The drawing under review shows one solid part. Ordinate dimensions are in mm from its lowest x, y, z. A direction names the side the tool comes from. Coordinates: 2 decimals unless noted, no trailing zeros. Write each loop counter-clockwise with the first axis right and the second up, starting at its lowest first coordinate (ties: lowest second). Pieces come first, ordered by that corner, then holes.
Q1. Add section C-C, the plane x = 5.5. Give the boundary of the cut face in (y, z), plus the area to 3 significant figures.
Q2. The part is to be moulded in two halves that separate along Z. For the marked faces 3, 4 and 5, say which applies: +Z half, -Z half, draft (parallel to the pull), parting line (faces both ways), or undercut.
Q3. Add section A-A, the plane z = 9. Give the boundary of the cut face in (x, y), plus the area to 3 significant figures.
Q4. Clearance check with flat-ended pins moving along their axes: pin 1 Ø3 at (x, y) = (6, 4) entering from +Z; pin 2 Ø2.5 at (y, z) = (9, 14.95) entering from +X; pin 3 Ø6.5 at (y, z) = (14.95, 9) entering from +X. State where each tip first meets the part, or that it passes through.
Q5. Add section D-D, the plane x = 1.25. Give the boundary of the cut face in (y, z).
Q6. Machinability: for the marked faces 1 and 2, which of the approach directions +Z, -Z, +X, -X, +Y, -Y give a long, thin tool a straight path to every point of the face, cutting with its end or side? Answer none if there is none.
Q7. To check wall thickness, follow probe 1 along Y at (x, z) = (5.75, 7.25); probe 2 along Z at (x, y) = (2.5, 10.25); probe 3 along Z at (x, y) = (4, 8.5). State the ranges of each line that lie inside material, in increasing order.
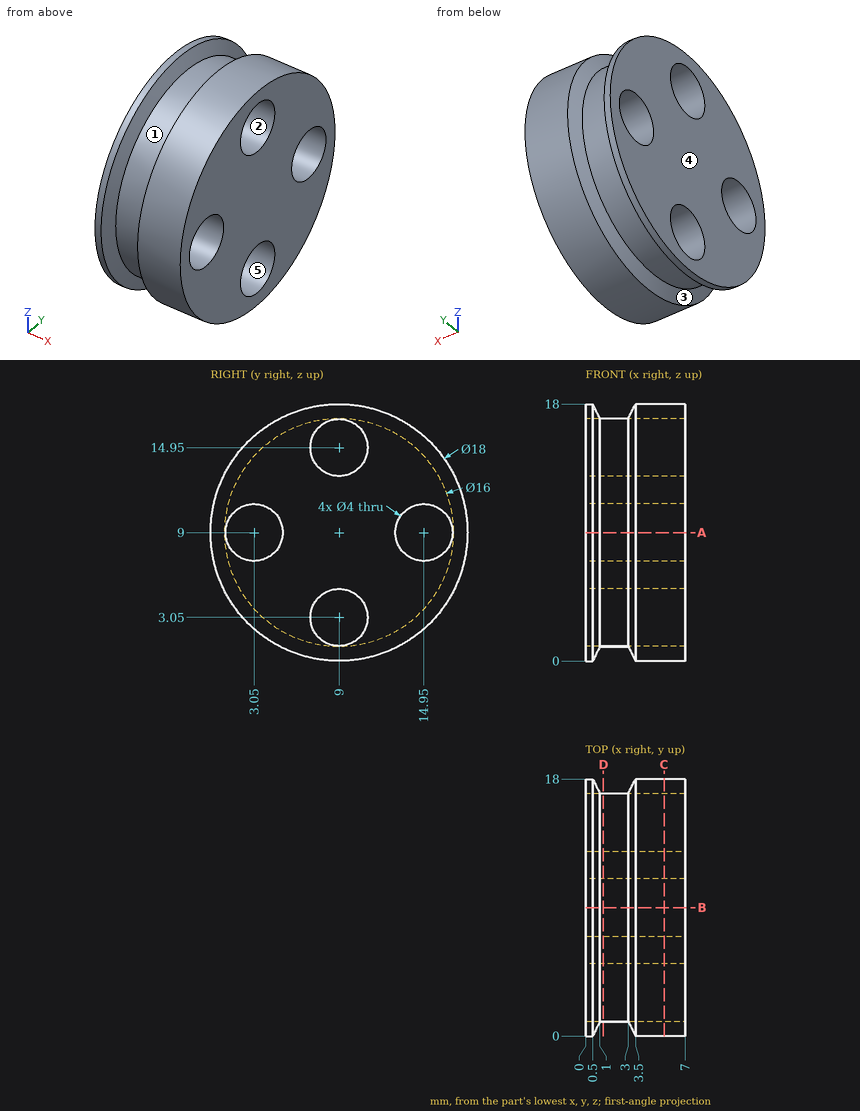
Here are the results:
1. outline: circle Ø18 at (9, 9); hole circle Ø4 at (3.05, 9); hole circle Ø4 at (9, 3.05); hole circle Ø4 at (9, 14.95); hole circle Ø4 at (14.95, 9)
1. area: 204 mm2
2. face 3: parting line
2. face 4: draft
2. face 5: undercut
3. outline: (0, 0) - (0.5, 0) - (1, 1) - (3, 1) - (3.5, 0) - (7, 0) - (7, 1.05) - (0, 1.05) - close; (0, 5.05) - (7, 5.05) - (7, 12.95) - (0, 12.95) - close; (0, 16.95) - (7, 16.95) - (7, 18) - (3.5, 18) - (3, 17) - (1, 17) - (0.5, 18) - (0, 18) - close
3. area: 65.0 mm2
4. pin 1: stops at z = 17.29
4. pin 2: passes through
4. pin 3: stops at x = 7
5. outline: circle Ø16 at (9, 9); hole circle Ø4 at (3.05, 9); hole circle Ø4 at (9, 3.05); hole circle Ø4 at (9, 14.95); hole circle Ø4 at (14.95, 9)
6. face 1: none
6. face 2: +X, -X
7. probe 1: y = 0.17 to 2.08, 4.02 to 13.98, 15.92 to 17.83
7. probe 2: z = 1.1 to 1.49, 4.61 to 13.39, 16.51 to 16.9
7. probe 3: z = 0.01 to 1.11, 4.99 to 13.01, 16.89 to 17.99
